Build history of the part. All positions in model axes, mm. Give positions to 0.01 mm unless a question says otherwise; leave off trailing zeros. Loops run counter-clockwise (first coordinate to the right, second up) from the corner with the lowest first, then second, coordinate; pieces in that order, holes last. Notation, with made-up numbers: M 43.5,0.5 L 50.5,0.5 A23 ccw 50.5,9.5 Z; hole C 9.5,75 d4. An arc over 180 degrees is marked long. Answer as a JSON object with one key per item and string values. Group by question number.
1. Drill centre lines: line 1 along X through (y, z) = (-12, 13); line 2 along Z through (x, y) = (3, -12); line 3 along Y through (x, z) = (-4.25, 23.5). Where is each one in solid material? Low to high. Write a range as [from, to].
2. Slice it at C-C (x = 6.5). List the corners of the cut face in (y, z), then the cut area to 3 significant figures.
3. Drop flat-ended pins along their axis: pin 1 Ø3 at (y, z) = (-11, 30) entering from +X; pin 2 Ø0.9 at (y, z) = (-10.5, 30.5) entering from -X; pin 3 Ø1 at (y, z) = (5.5, 30) entering from -X. Give the stop position or say it passes through.
4. Slice it at A-A (z = 34). List the corners of the cut face in (x, y).
5. Slice it at B-B (y = -10.25). List the corners of the cut face in (x, z).
from build123d import *

# Parameters (mm, degrees)
F1_DEPTH    = 50.8
F2_R        = 2
F3_R        = 5
F4_T1_DEPTH = 23


# Not quite as in the source:
# - a fillet or chamfer that OpenCascade refuses, or shapes differently, is made with other operations: its cross-section is extruded or revolved along the edge and cut away or added


with BuildPart() as f1:
    # F0 (on Top) → F1 (new body)
    with BuildSketch(Plane.XY):
        with BuildLine():
            ThreePointArc((6, -7.3008561142), (8.5440768957, -4.0374806501), (9.45, 0))
            ThreePointArc((9.45, 0), (-4.0374806501, 8.5440768957), (-6, -7.3008561142))
            ThreePointArc((-6, -7.3008561142), (0, -9.45), (6, -7.3008561142))
        make_face()
        with BuildLine():
            ThreePointArc((6, -7.3008561142), (0, -9.45), (-6, -7.3008561142))
            Line((-6, -7.3008561142), (-6, -14.3008561142))
            Line((-6, -14.3008561142), (0, -14.3008561142))
            Line((0, -14.3008561142), (6, -14.3008561142))
            Line((6, -14.3008561142), (6, -7.3008561142))
        make_face()
    extrude(amount=F1_DEPTH)

    # F2
    f2_edges = [f1.edges().sort_by_distance(p)[0] for p in [
        (6, -14.300856, 25.4),
        (-6, -14.300856, 25.4),
    ]]
    fillet(f2_edges, radius=F2_R)

    # F3
    f3_edges = [f1.edges().sort_by_distance(p)[0] for p in [
        (-6, -7.300856, 25.4),
        (6, -7.300856, 25.4),
    ]]
    fillet(f3_edges, radius=F3_R)

    # F4: fillet of radius 3 on 1 edges, made by hand

    # F4_s2 → F4_t1 (cut)
    with BuildSketch(Plane.YZ.offset(-11.5)):
        with BuildLine():
            ThreePointArc((-11.3008561142, 50.8), (-13.4221764577, 49.9213203436), (-14.3008561142, 47.8))
            Line((-14.3008561142, 47.8), (-14.3008561142, 50.8))
            Line((-14.3008561142, 50.8), (-11.3008561142, 50.8))
        make_face()
    extrude(amount=F4_T1_DEPTH, mode=Mode.SUBTRACT)


solid = f1.part
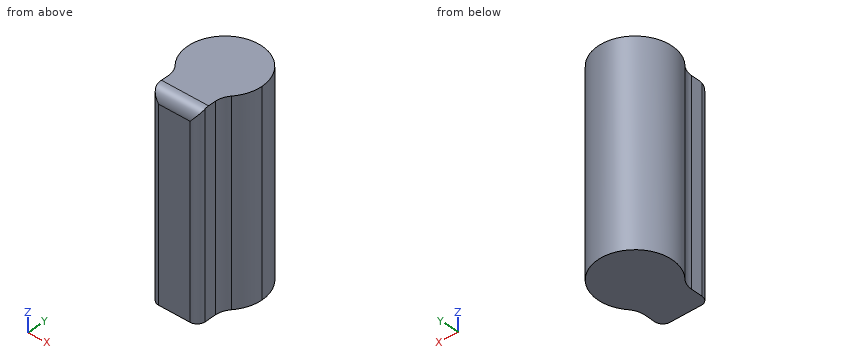
Established:
{
 "1": {"line 1": "x = [-6, 6]", "line 2": "z = [0, 50.72]", "line 3": "y = [-14.29, 8.44]"},
 "2": {"outline": "M -7.19,0 L 6.86,0 L 6.86,50.8 L -7.19,50.8 Z", "area": "714 mm^2"},
 "3": {"pin 1": "stops at x = 6", "pin 2": "stops at x = -6", "pin 3": "stops at x = -8.02"},
 "4": {"outline": "M -7.19,-6.13 A5 cw -6,-9.37 L -6,-12.3 A2 ccw -4,-14.3 L 4,-14.3 A2 ccw 6,-12.3 L 6,-9.37 A5 cw 7.19,-6.13 A9.45 ccw long Z"},
 "5": {"outline": "M -6,0 L 6,0 L 6,50.8 L -6,50.8 Z"}
}
